Could you check a few things on this drawing? It's one solid part, dimensions in mm from its lowest x, y, z. A direction names the side the tool comes from. Coordinates: 2 decimals unless noted, no trailing zeros. Write each loop counter-clockwise with the first axis right and the second up, starting at its lowest first coordinate (ties: lowest second). Pieces come first, ordered by that corner, then holes.
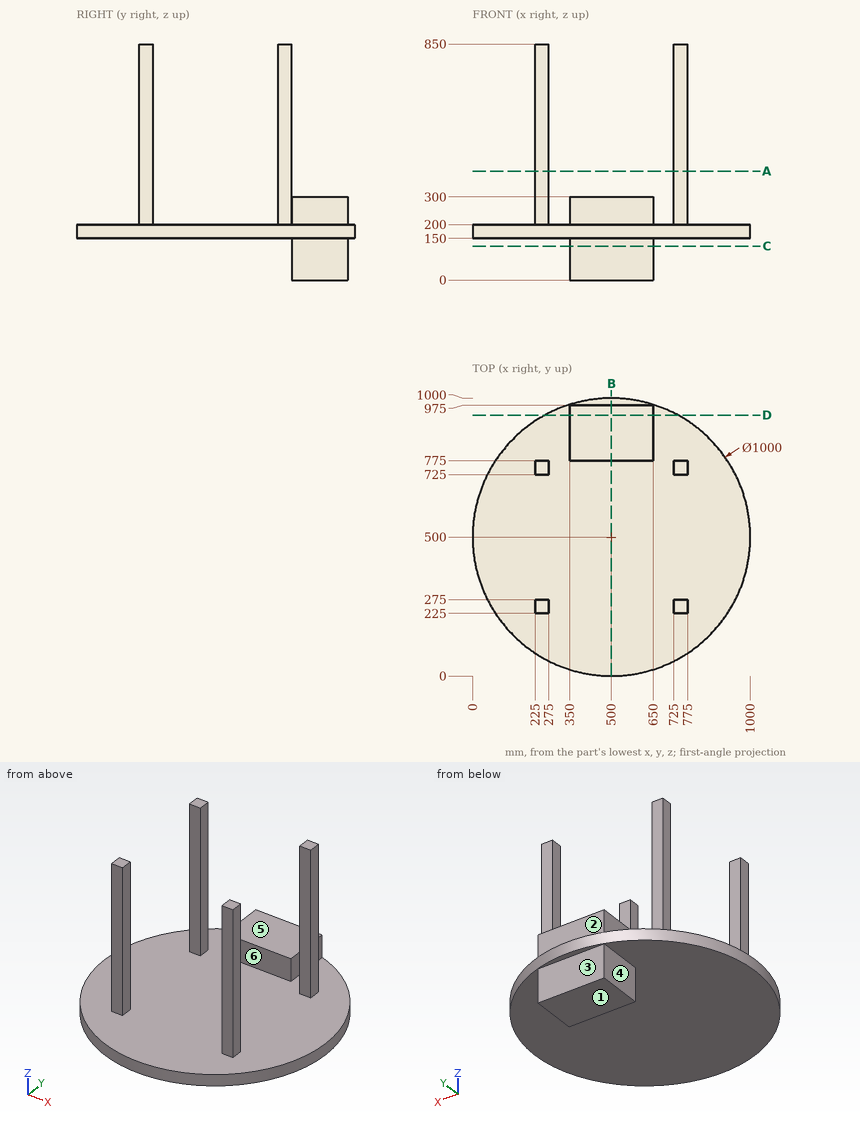
1) On a 3-axis mill with a long thin cutter (end or side, diameter ignored), from which of +Z, -Z, +X, -X, +Y, -Y can I reach the whole of each face in a straight line? I mean the marked faces 1, 2 and 3. Say none if no direction works.
Values follow:
face 1: -Z, +X, -X, +Y, -Y
face 2: +Z, +X, -X, +Y
face 3: -Z, +X, -X, +Y
2) Imagine slicing it at A-A on z = 392. Please give me the cut outline in (x, y).
Values follow:
outline: (225, 225) - (275, 225) - (275, 275) - (225, 275) - close; (225, 725) - (275, 725) - (275, 775) - (225, 775) - close; (725, 225) - (775, 225) - (775, 275) - (725, 275) - close; (725, 725) - (775, 725) - (775, 775) - (725, 775) - close
3) We'd pull the mould along X, two halves only. Please class the marked faces 4, 5 and 6: pulls with the +X half, pulls with the -X half, needs draft (parallel to the pull), parting line crosses it, or undercut.
Values follow:
face 4: pulls with the -X half
face 5: needs draft
face 6: undercut
4) Imagine slicing it at B-B on x = 500. Please give me the cut outline in (y, z).
Values follow:
outline: (0, 150) - (775, 150) - (775, 0) - (975, 0) - (975, 150) - (1000, 150) - (1000, 200) - (975, 200) - (975, 300) - (775, 300) - (775, 200) - (0, 200) - close
5) Imagine slicing it at C-C on z = 122.5. Please give me the cut outline in (x, y).
Values follow:
outline: (350, 775) - (650, 775) - (650, 975) - (350, 975) - close
6) Will these pins go through, and if not, where does the flat tip stop? pin 1 (12 mm diameter, centred on x = 143.5, y = 449.5, fed in from -Z); pin 2 (2 mm diameter, centred on x = 630.5, z = 138, fed in from +Y); pin 3 (15 mm diameter, centred on y = 250, z = 634.5, fed in from +X).
Values follow:
pin 1: stops at z = 150
pin 2: stops at y = 975
pin 3: stops at x = 775
7) I need wall thicknesses on probe 1 along X at (y, z) = (941.5, 264); probe 2 along Z at (x, y) = (508.5, 830); probe 3 along Z at (x, y) = (295, 532). Which ranges of each line are inside material? Lowest first, please.
Values follow:
probe 1: x = 350 to 650
probe 2: z = 0 to 300
probe 3: z = 150 to 200
8) Imagine slicing it at D-D on y = 939. Please give me the cut outline in (x, z), then the cut area to 3 significant figures.
Values follow:
outline: (260.67, 150) - (350, 150) - (350, 0) - (650, 0) - (650, 150) - (739.33, 150) - (739.33, 200) - (650, 200) - (650, 300) - (350, 300) - (350, 200) - (260.67, 200) - close
area: 98,900 mm2
